The listing builds one solid part. Answer for the finished solid, in the listing's coordinates (mm). Round coordinates to 2 decimals unless told otherwise and drop trailing zeros. Loops run counter-clockwise (first coordinate to the right, second up) from the corner with the lowest first, then second, coordinate; pieces in that order, holes last. Notation, with made-up numbers: (82, 77.25) -> (90, 77.25) arc R15 ccw to (90, 91.25) -> close; hole circle Ø6 at (85, -30.5). An arc over 180 degrees is marked (long way). One line per question, with ' | ' between items.
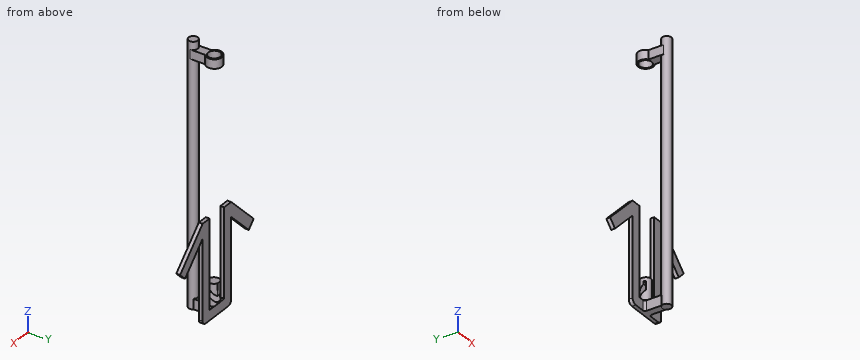
from build123d import *

# Parameters (mm, degrees)
SKETCH1_R               = 3
BOSS_EXTRUDE1_DEPTH     = 170
SKETCH3_W               = 4.850977856
SKETCH3_H               = 6.691139058
BOSS_EXTRUDE2_DEPTH     = 13
SKETCH5_W               = 14
SKETCH5_H               = 6.691139058
BOSS_EXTRUDE4_DEPTH     = 2.5
FILLET1_R               = 1.5
FILLET2_R               = 3
BOSS_EXTRUDE6_DEPTH     = 14.5
FILLET3_R               = 3
CUT_EXTRUDE1_DEPTH      = 4
CUT_EXTRUDE1_DEPTH_BACK = 4.5
SKETCH15_W              = 6
SKETCH15_H              = 5.998501846
BOSS_EXTRUDE7_DEPTH     = 16.843139176
SKETCH16_R              = 5
SKETCH16_R_2            = 4
BOSS_EXTRUDE9_DEPTH     = 5.998501846
CUT_EXTRUDE6_START      = -5.998501846
SKETCH17_R              = 4
CUT_EXTRUDE6_DEPTH      = 5.998501846


with BuildPart() as part:
    # Sketch1 → Boss-Extrude1 (new body)
    with BuildSketch(Plane.XY):
        Circle(SKETCH1_R)
    extrude(amount=BOSS_EXTRUDE1_DEPTH)

    # Sketch3 → Boss-Extrude2 (add)
    with BuildSketch(Plane(origin=(0, 0, 0), x_dir=(1, 0, 0), z_dir=(0, 1, 0))):
        with Locations((0, -3.488992019)):
            Rectangle(SKETCH3_W, SKETCH3_H)
    extrude(amount=BOSS_EXTRUDE2_DEPTH)

    # Sketch5 → Boss-Extrude4 (add)
    with BuildSketch(Plane(origin=(0, 13, 0), x_dir=(1, 0, 0), z_dir=(0, 1, 0))):
        with Locations((0, -3.488992019)):
            Rectangle(SKETCH5_W, SKETCH5_H)
        Polygon((-7, -6.834561548), (-7, -0.14342249), (-13.7, -0.14342249), (-13.7, -55.421203077), (-30.531042429, -38.590160648), (-35.268657863, -43.327776082), (-13.7, -64.896433945), (-7, -64.896433945), align=None)
        Polygon((13.7, -0.14342249), (7, -0.14342249), (7, -6.834561548), (7, -64.896433945), (13.7, -64.896433945), (35.268657863, -43.327776082), (30.531042429, -38.590160648), (13.7, -55.421203077), align=None)
    extrude(amount=BOSS_EXTRUDE4_DEPTH)

    # Fillet1
    fillet1_edges = [part.edges().sort_by_distance(p)[0] for p in [
        (-2.425488928, 13, 3.488992019),
        (2.425488928, 13, 3.488992019),
    ]]
    fillet(fillet1_edges, radius=FILLET1_R)

    # Fillet2
    fillet2_edges = [part.edges().sort_by_distance(p)[0] for p in [
        (13.7, 14.25, 0.14342249),
        (-13.7, 14.25, 0.14342249),
    ]]
    fillet(fillet2_edges, radius=FILLET2_R)

    # Sketch8 → Boss-Extrude6 (add)
    with BuildSketch(Plane.XY.offset(6.834561548)):
        with BuildLine():
            Line((-1.341226683, 16.843139176), (1.341226683, 16.843139176))
            ThreePointArc((1.341226683, 16.843139176), (0, 10.260613318), (-1.341226683, 16.843139176))
        make_face()
    extrude(amount=BOSS_EXTRUDE6_DEPTH)

    # Fillet3
    # the kernel refuses this fillet: 3 mm, written as the material it takes off along each edge
    with BuildSketch(Plane(origin=(-7.593632325, 16.843139176, 6.834561548), x_dir=(0, -1.0, 1.7735276910753176e-12), z_dir=(1, 0, 0))) as fillet3_piece_1:
        with BuildLine():
            CenterArc((3, -2.500962257), FILLET3_R, 123.524048603, 56.475951397)
            Line((0, -2.500962257), (-0.06, -2.500962257))
            Line((-0.06, -2.500962257), (-0.06, 0))
            Line((-0.06, 0), (0, 0.06))
            ThreePointArc((0, 0.06), (0.671569588, 0.06), (1.31000196, 0.050019245))
            Line((1.31000196, 0.050019245), (1.343139176, 0))
        make_face()
    extrude(amount=15.187264651, mode=Mode.SUBTRACT)

    # Sketch14 → Cut-Extrude1 (cut, two sides: drawn at the far end of the back side and taken through both)
    with BuildSketch(Plane(origin=(0, 0, 0), x_dir=(0, 0, -1), z_dir=(1, 0, 0)).offset(-CUT_EXTRUDE1_DEPTH_BACK)):
        Polygon((-9.335523805, 16.843139176), (-13.335523805, 16.843139176), (-17.161439006, 12.918121422), (-19.074284697, 12.918121422), (-19.074284697, 11.627222293), (-13.335523805, 11.627222293), align=None)
    extrude(amount=CUT_EXTRUDE1_DEPTH + CUT_EXTRUDE1_DEPTH_BACK, mode=Mode.SUBTRACT)

    # Sketch15 → Boss-Extrude7 (add)
    with BuildSketch(Plane(origin=(0, 0, 0), x_dir=(1, 0, 0), z_dir=(0, 1, 0))):
        with Locations((0, -161.824268897)):
            Rectangle(SKETCH15_W, SKETCH15_H)
    extrude(amount=BOSS_EXTRUDE7_DEPTH)

    # Sketch16 → Boss-Extrude9 (add)
    with BuildSketch(Plane(origin=(0, 0, 158.825017974), x_dir=(-1, 0, 0), z_dir=(0, 0, -1))):
        with Locations((0, 13.803369952)):
            Circle(SKETCH16_R)
        with Locations((0, 13.803369952)):
            Circle(SKETCH16_R_2, mode=Mode.SUBTRACT)
    extrude(amount=-BOSS_EXTRUDE9_DEPTH)

    # Sketch17 → Cut-Extrude6 (cut)
    with BuildSketch(Plane.XY.offset(164.82351982).offset(CUT_EXTRUDE6_START)):
        with Locations(Location((0, 13.803369952, 0), (0, 0, 180))):
            Circle(SKETCH17_R)
    extrude(amount=CUT_EXTRUDE6_DEPTH, mode=Mode.SUBTRACT)


solid = part.part
Q1. Find the intervals of material crossed by line 1 (Y direction, x = 0, z = 160.8); line 2 (X direction, y = 13.5, z = 60.5); line 3 (Z direction, x = 10, y = 13.75), in increasing order. Write a range as from..to.
Numbers:
line 1: -3..9.8, 17.8..18.8 | line 2: -18.1..-7, 7..18.1 | line 3: 0.14..64.9
Q2. A cutting plane is placed at B-B on x = -28. Give the vertices of the cut face in (y, z).
Numbers:
outline: (13, 41.12) -> (15.5, 41.12) -> (15.5, 50.6) -> (13, 50.6) -> close
Q3. Given pin 1 Ø7 at (x, y) = (1, 10.5) entering from -Z; pin 2 Ø12 at (y, z) = (16.5, 54) entering from -X; pin 3 Ø0.8 at (x, z) = (0, 18.5) entering from +Y, each flat-ended and moving along its own axis, determine where each tip first touches the part or whether it passes through.
Numbers:
pin 1: z = 0.14 | pin 2: x = -30.51 | pin 3: y = 16.84
Q4. A cutting plane is placed at A-A on y = 5.5. Give the vertices of the cut face in (x, z).
Numbers:
outline: (-3, 158.83) -> (3, 158.83) -> (3, 164.82) -> (-3, 164.82) -> close; (-2.43, 0.14) -> (2.43, 0.14) -> (2.43, 6.83) -> (-2.43, 6.83) -> close
